Model file for the job. Use its own axes, mm. Face numbers are marked on the shaded views. A direction names the side the tool comes from. Coordinates: 2 decimals unless noted, no trailing zeros. Write each loop counter-clockwise with the first axis right and the second up, starting at its lowest first coordinate (ties: lowest second). Pieces come first, ordered by that corner, then holes. Notation, with made-up numbers: M 83,18.5 L 118,18.5 A19 ccw 118,27.5 Z; hole C 29,-12.5 d2. An arc over 180 degrees is marked long. One line per question, with ' | ' between items. Start each with the question number.
(1) Wall check: probe 1 along Z at (x, y) = (0, 2.25); probe 2 along Z at (x, y) = (0, 3.95); probe 3 along Z at (x, y) = (7, 6.5). Give the ranges that are in metal, low to high.
(2) Cut at D-D (x = -3.25). Write the cut outline in (y, z).
(3) Cut at B-B (z = -11.25). Write the cut outline in (x, y), plus the area to 3 significant figures.
(4) Two-plate mould, pull along X, no slides. Class the marked faces 4, 5 and 6: +X half, -X half, draft (parallel to the pull), parting line (faces both ways), or undercut.
(5) Flat gauge pins, fed straight in: pin 1 Ø3.5 at (x, z) = (-8, 7.5) entering from +Y; pin 2 Ø1 at (x, y) = (8.5, 6.5) entering from -Z; pin 3 Ø4 at (x, z) = (0, 11.11) entering from +Y; pin 4 Ø7.5 at (x, z) = (1, 3.5) entering from -Y. Where does each tip first touch, or does it go through?
(6) Cut at C-C (y = 7.25). Write the cut outline in (x, z) (1 decimal), plus the area to 3 significant figures.
(7) Tool access for the marked faces 1, 2 and 3: list every direction of +Z, -Z, +X, -X, +Y, -Y with a clear straight run to the whole face (end or side of a thin tool).
(8) Cut at A-A (x = 0). Write the cut outline in (y, z).
Autodesk Inventor part; units mm, degrees
ref_plane "a1_XY" through (0, 8.7376, -14.1351) normal (0, 1, 0) x (1, 0, 0)
ref_plane "a1_YZ" through (0, 8.7376, -14.1351) normal (1, 0, 0) x (0, 0, -1)
ref_plane "a1_ZX" through (0, 8.7376, -14.1351) normal (0, 0, -1) x (0, 1, 0)
sketch "Sketch_1" plane through (0, 0, 0) normal (0, 0, 1) x (1, 0, 0)
  line L0 (0, 0) -> (0, 8.7376)
  line L1 (0, 8.7376) -> (14.1351, 8.7376)
  line L2 (14.1351, 8.7376) -> (14.1351, 0)
  line L3 (14.1351, 0) -> (0, 0)
  line L4 (0, 0) -> (0, 8.7376)
revolve "Revolution1" add sketch "Sketch_1" angle 360 about axis through (0, 0, 0) along (0, -1, 0)
sketch "Sketch_63" plane through (0, 0, 0) normal (0, 1, 0) x (-1, 0, 0)
  line L0 (20.6184, 14.1351) -> (13.5509, 14.1351)
  line L1 (13.5509, 14.1351) -> (13.5509, -14.1351)
  line L2 (13.5509, -14.1351) -> (20.6184, -14.1351)
  line L3 (20.6184, -14.1351) -> (20.6184, 14.1351)
extrude "Extrusion1" cut sketch "Sketch_63" along normal blind 8.7376
sketch "Sketch_37" plane through (0, 0, 0) normal (0, 0, 1) x (1, 0, 0)
  line L0 (-5.8778, 4.3688) -> (-14.1351, 4.3688)
  line L1 (-14.1351, 4.3688) -> (-14.1351, 8.3376)
  line L2 (-14.1351, 8.3376) -> (-13.5509, 8.3376)
  line L3 (-13.5509, 8.3376) -> (-13.5509, 6.7818)
  line L4 (-13.5509, 6.7818) -> (-13.1216, 6.3525)
  line L5 (-13.1216, 6.3525) -> (-7.0231, 6.3525)
  line L6 (-7.0231, 6.3525) -> (-5.8778, 4.3688)
  line L7 (-5.8778, 4.3688) -> (-14.1351, 4.3688)
revolve "Revolution2" cut sketch "Sketch_37" angle 360 about axis through (-5.8778, 4.3688, 0) along (1, 0, 0)
thread "Thread1"
sketch "Sketch4" plane through (0, 0, 0) normal (0, -1, 0) x (1, 0, 0)
  point P0 (0, 0)
hole "Hole1" at (0, 0, 0) direction (0, 1, 0) diameter 15.494 depth 2.54
sketch "Sketch5" plane through (0, 8.7376, 0) normal (0, 1, 0) x (1, 0, 0)
  point P0 (0, -11.1125)
hole "Hole2" at (0, 8.7376, 11.1125) direction (0, -1, 0) diameter 3.2639 depth 8.7376 counterbore diameter 4.953 counterbore depth 3.048
sketch "Sketch6" plane through (0, 8.7376, 0) normal (0, 1, 0) x (1, 0, 0)
  point P0 (0, 11.1125)
hole "Hole3" at (0, 8.7376, -11.1125) direction (0, -1, 0) diameter 3.2639 depth 8.7376 counterbore diameter 4.953 counterbore depth 3.048
sketch "Sketch7" plane through (0, 8.7376, 0) normal (0, 1, 0) x (1, 0, 0)
  point P0 (-7.7589, -7.7589)
hole "Hole4" at (-7.7589, 8.7376, 7.7589) direction (0, -1, 0) diameter 2.1565 depth 8.7376 counterbore diameter 3.048 counterbore depth 2.54
pattern_linear "Rectangular Pattern1" count 2 spacing 15.5179 along (1, 0, 0) count 2 spacing 15.5179 along (0, 0, -1) of "Hole4"
ref_plane "a1_XY" through (0, 8.7376, -14.1351) normal (0, 1, 0) x (1, 0, 0)
ref_plane "a1_YZ" through (0, 8.7376, -14.1351) normal (1, 0, 0) x (0, 0, -1)
ref_plane "a1_ZX" through (0, 8.7376, -14.1351) normal (0, 0, -1) x (0, 1, 0)
ref_plane "a2_XY" through (0, 8.7376, 14.1351) normal (0, 1, 0) x (1, 0, 0)
ref_plane "a2_YZ" through (0, 8.7376, 14.1351) normal (1, 0, 0) x (0, 0, -1)
ref_plane "a2_ZX" through (0, 8.7376, 14.1351) normal (0, 0, -1) x (0, 1, 0)
ref_plane "ar3_XY" through (-7.9026, 2.54, 7.9026) normal (0, 1, 0) x (1, 0, 0)
ref_plane "ar3_YZ" through (-7.9026, 2.54, 7.9026) normal (1, 0, 0) x (0, 0, -1)
ref_plane "ar3_ZX" through (-7.9026, 2.54, 7.9026) normal (0, 0, -1) x (0, 1, 0)
ref_plane "ar4_XY" through (7.9026, 2.54, 7.9026) normal (0, 1, 0) x (1, 0, 0)
ref_plane "ar4_YZ" through (7.9026, 2.54, 7.9026) normal (1, 0, 0) x (0, 0, -1)
ref_plane "ar4_ZX" through (7.9026, 2.54, 7.9026) normal (0, 0, -1) x (0, 1, 0)
ref_plane "ar5_XY" through (7.9026, 2.54, -7.9026) normal (0, 1, 0) x (1, 0, 0)
ref_plane "ar5_YZ" through (7.9026, 2.54, -7.9026) normal (1, 0, 0) x (0, 0, -1)
ref_plane "ar5_ZX" through (7.9026, 2.54, -7.9026) normal (0, 0, -1) x (0, 1, 0)
ref_plane "ar6_XY" through (-7.9026, 2.54, -7.9026) normal (0, 1, 0) x (1, 0, 0)
ref_plane "ar6_YZ" through (-7.9026, 2.54, -7.9026) normal (1, 0, 0) x (0, 0, -1)
ref_plane "ar6_ZX" through (-7.9026, 2.54, -7.9026) normal (0, 0, -1) x (0, 1, 0)
ref_plane "b1_XY" through (0, 8.7376, 0) normal (0, 1, 0) x (1, 0, 0)
ref_plane "b1_YZ" through (0, 8.7376, 0) normal (1, 0, 0) x (0, 0, -1)
ref_plane "b1_ZX" through (0, 8.7376, 0) normal (0, 0, -1) x (0, 1, 0)
ref_plane "j_XY" through (0, 0, 0) normal (0, 1, 0) x (1, 0, 0)
ref_plane "j_YZ" through (0, 0, 0) normal (1, 0, 0) x (0, 0, -1)
ref_plane "j_ZX" through (0, 0, 0) normal (0, 0, -1) x (0, 1, 0)
ref_plane "k1_XY" through (-13.5509, 4.3688, 0) normal (0, 0, 1) x (1, 0, 0)
ref_plane "k1_YZ" through (-13.5509, 4.3688, 0) normal (1, 0, 0) x (0, 1, 0)
ref_plane "k1_ZX" through (-13.5509, 4.3688, 0) normal (0, 1, 0) x (0, 0, 1)
ref_plane "k2_XY" through (-13.5509, 8.7376, 0) normal (0, 0, 1) x (1, 0, 0)
ref_plane "k2_YZ" through (-13.5509, 8.7376, 0) normal (1, 0, 0) x (0, 1, 0)
ref_plane "k2_ZX" through (-13.5509, 8.7376, 0) normal (0, 1, 0) x (0, 0, 1)
ref_plane "l1_XY" through (-13.5509, 6.7818, 0) normal (0, 0, 1) x (1, 0, 0)
ref_plane "l1_YZ" through (-13.5509, 6.7818, 0) normal (1, 0, 0) x (0, 1, 0)
ref_plane "l1_ZX" through (-13.5509, 6.7818, 0) normal (0, 1, 0) x (0, 0, 1)
ref_plane "l2_XY" through (-13.5509, 1.9558, 0) normal (0, 0, 1) x (1, 0, 0)
ref_plane "l2_YZ" through (-13.5509, 1.9558, 0) normal (1, 0, 0) x (0, 1, 0)
ref_plane "l2_ZX" through (-13.5509, 1.9558, 0) normal (0, 1, 0) x (0, 0, 1)
ref_plane "po1_XY" through (10.9728, 0, 0) normal (0, 1, 0) x (1, 0, 0)
ref_plane "po1_YZ" through (10.9728, 0, 0) normal (1, 0, 0) x (0, 0, -1)
ref_plane "po1_ZX" through (10.9728, 0, 0) normal (0, 0, -1) x (0, 1, 0)
ref_plane "po2_XY" through (-5.4864, 0, -9.5027) normal (0, 1, 0) x (1, 0, 0)
ref_plane "po2_YZ" through (-5.4864, 0, -9.5027) normal (1, 0, 0) x (0, 0, -1)
ref_plane "po2_ZX" through (-5.4864, 0, -9.5027) normal (0, 0, -1) x (0, 1, 0)
ref_plane "po3_XY" through (-5.4864, 0, 9.5027) normal (0, 1, 0) x (1, 0, 0)
ref_plane "po3_YZ" through (-5.4864, 0, 9.5027) normal (1, 0, 0) x (0, 0, -1)
ref_plane "po3_ZX" through (-5.4864, 0, 9.5027) normal (0, 0, -1) x (0, 1, 0)
ref_plane "r7_XY" through (-1.7526, 8.7376, -11.1125) normal (0, 1, 0) x (1, 0, 0)
ref_plane "r7_YZ" through (-1.7526, 8.7376, -11.1125) normal (1, 0, 0) x (0, 0, -1)
ref_plane "r7_ZX" through (-1.7526, 8.7376, -11.1125) normal (0, 0, -1) x (0, 1, 0)
ref_plane "r71_XY" through (0, 8.7376, 11.1125) normal (0, 1, 0) x (1, 0, 0)
ref_plane "r71_YZ" through (0, 8.7376, 11.1125) normal (1, 0, 0) x (0, 0, -1)
ref_plane "r71_ZX" through (0, 8.7376, 11.1125) normal (0, 0, -1) x (0, 1, 0)
ref_plane "r72_XY" through (1.7526, 8.7376, -11.1125) normal (0, 1, 0) x (1, 0, 0)
ref_plane "r72_YZ" through (1.7526, 8.7376, -11.1125) normal (1, 0, 0) x (0, 0, -1)
ref_plane "r72_ZX" through (1.7526, 8.7376, -11.1125) normal (0, 0, -1) x (0, 1, 0)
ref_plane "r73_XY" through (0, 8.7376, -11.1125) normal (0, 1, 0) x (1, 0, 0)
ref_plane "r73_YZ" through (0, 8.7376, -11.1125) normal (1, 0, 0) x (0, 0, -1)
ref_plane "r73_ZX" through (0, 8.7376, -11.1125) normal (0, 0, -1) x (0, 1, 0)
ref_plane "rg_XY" through (0, 8.7376, 0) normal (0, 1, 0) x (1, 0, 0)
ref_plane "rg_YZ" through (0, 8.7376, 0) normal (1, 0, 0) x (0, 0, -1)
ref_plane "rg_ZX" through (0, 8.7376, 0) normal (0, 0, -1) x (0, 1, 0)
ref_plane "rh_XY" through (0, 8.7376, 0) normal (0, 1, 0) x (1, 0, 0)
ref_plane "rh_YZ" through (0, 8.7376, 0) normal (1, 0, 0) x (0, 0, -1)
ref_plane "rh_ZX" through (0, 8.7376, 0) normal (0, 0, -1) x (0, 1, 0)
ref_plane "rs_1_XY" through (0, 10.5156, -11.1125) normal (0, 1, 0) x (1, 0, 0)
ref_plane "rs_1_YZ" through (0, 10.5156, -11.1125) normal (1, 0, 0) x (0, 0, -1)
ref_plane "rs_1_ZX" through (0, 10.5156, -11.1125) normal (0, 0, -1) x (0, 1, 0)
ref_plane "rs_2_XY" through (-11.1125, 10.5156, 0) normal (0, 1, 0) x (1, 0, 0)
ref_plane "rs_2_YZ" through (-11.1125, 10.5156, 0) normal (1, 0, 0) x (0, 0, -1)
ref_plane "rs_2_ZX" through (-11.1125, 10.5156, 0) normal (0, 0, -1) x (0, 1, 0)
ref_plane "rs_3_XY" through (0, 10.5156, 11.1125) normal (0, 1, 0) x (1, 0, 0)
ref_plane "rs_3_YZ" through (0, 10.5156, 11.1125) normal (1, 0, 0) x (0, 0, -1)
ref_plane "rs_3_ZX" through (0, 10.5156, 11.1125) normal (0, 0, -1) x (0, 1, 0)
ref_plane "rs_4_XY" through (11.1125, 10.5156, 0) normal (0, 1, 0) x (1, 0, 0)
ref_plane "rs_4_YZ" through (11.1125, 10.5156, 0) normal (1, 0, 0) x (0, 0, -1)
ref_plane "rs_4_ZX" through (11.1125, 10.5156, 0) normal (0, 0, -1) x (0, 1, 0)
ref_plane "sc1_XY" through (10.9728, 4.9276, 0) normal (0, 1, 0) x (1, 0, 0)
ref_plane "sc1_YZ" through (10.9728, 4.9276, 0) normal (1, 0, 0) x (0, 0, -1)
ref_plane "sc1_ZX" through (10.9728, 4.9276, 0) normal (0, 0, -1) x (0, 1, 0)
ref_plane "sc2_XY" through (-5.4864, 4.9276, -9.5027) normal (0, 1, 0) x (1, 0, 0)
ref_plane "sc2_YZ" through (-5.4864, 4.9276, -9.5027) normal (1, 0, 0) x (0, 0, -1)
ref_plane "sc2_ZX" through (-5.4864, 4.9276, -9.5027) normal (0, 0, -1) x (0, 1, 0)
ref_plane "sc3_XY" through (-5.4864, 4.9276, 9.5027) normal (0, 1, 0) x (1, 0, 0)
ref_plane "sc3_YZ" through (-5.4864, 4.9276, 9.5027) normal (1, 0, 0) x (0, 0, -1)
ref_plane "sc3_ZX" through (-5.4864, 4.9276, 9.5027) normal (0, 0, -1) x (0, 1, 0)
ref_plane "to_dummy_XY" through (0, 8.7376, 0) normal (0, 1, 0) x (1, 0, 0)
ref_plane "to_dummy_YZ" through (0, 8.7376, 0) normal (1, 0, 0) x (0, 0, -1)
ref_plane "to_dummy_ZX" through (0, 8.7376, 0) normal (0, 0, -1) x (0, 1, 0)
ref_plane "to_nut_XY" through (0, 10.2616, 0) normal (0, 1, 0) x (1, 0, 0)
ref_plane "to_nut_YZ" through (0, 10.2616, 0) normal (1, 0, 0) x (0, 0, -1)
ref_plane "to_nut_ZX" through (0, 10.2616, 0) normal (0, 0, -1) x (0, 1, 0)
ref_plane "to_rod_XY" through (0, 8.7376, 0) normal (0, 1, 0) x (1, 0, 0)
ref_plane "to_rod_YZ" through (0, 8.7376, 0) normal (1, 0, 0) x (0, 0, -1)
ref_plane "to_rod_ZX" through (0, 8.7376, 0) normal (0, 0, -1) x (0, 1, 0)
ref_plane "to_tube_XY" through (0, 2.54, 0) normal (0, 1, 0) x (1, 0, 0)
ref_plane "to_tube_YZ" through (0, 2.54, 0) normal (1, 0, 0) x (0, 0, -1)
ref_plane "to_tube_ZX" through (0, 2.54, 0) normal (0, 0, -1) x (0, 1, 0)
ref_plane "to_wiper_XY" through (0, 8.7376, 0) normal (0, 1, 0) x (1, 0, 0)
ref_plane "to_wiper_YZ" through (0, 8.7376, 0) normal (1, 0, 0) x (0, 0, -1)
ref_plane "to_wiper_ZX" through (0, 8.7376, 0) normal (0, 0, -1) x (0, 1, 0)
ref_plane "track1_XY" through (-7.7851, 0, 0) normal (0, 1, 0) x (1, 0, 0)
ref_plane "track1_YZ" through (-7.7851, 0, 0) normal (1, 0, 0) x (0, 0, -1)
ref_plane "track1_ZX" through (-7.7851, 0, 0) normal (0, 0, -1) x (0, 1, 0)
ref_plane "track2_XY" through (0, 0, -7.7851) normal (0, 1, 0) x (1, 0, 0)
ref_plane "track2_YZ" through (0, 0, -7.7851) normal (1, 0, 0) x (0, 0, -1)
ref_plane "track2_ZX" through (0, 0, -7.7851) normal (0, 0, -1) x (0, 1, 0)
ref_plane "track3_XY" through (7.7851, 0, 0) normal (0, 1, 0) x (1, 0, 0)
ref_plane "track3_YZ" through (7.7851, 0, 0) normal (1, 0, 0) x (0, 0, -1)
ref_plane "track3_ZX" through (7.7851, 0, 0) normal (0, 0, -1) x (0, 1, 0)
ref_plane "track4_XY" through (0, 0, 7.7851) normal (0, 1, 0) x (1, 0, 0)
ref_plane "track4_YZ" through (0, 0, 7.7851) normal (1, 0, 0) x (0, 0, -1)
ref_plane "track4_ZX" through (0, 0, 7.7851) normal (0, 0, -1) x (0, 1, 0)
properties part number "02-2-0.125-FO1_BM_heads_left-bif"
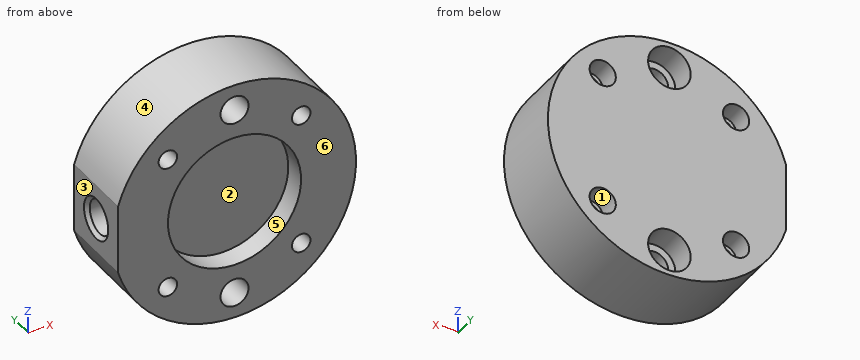
Filled in:
1) probe 1: -14.14 to -12.74, -9.48 to -7.75, 7.75 to 9.48, 12.74 to 14.14 | probe 2: -14.14 to -12.74, -9.48 to 9.48, 12.74 to 14.14 | probe 3: -12.28 to -9.08, -6.44 to 6.44, 9.08 to 12.28
2) outline: M 0,-13.76 L 8.74,-13.76 L 8.74,13.76 L 0,13.76 L 0,7.03 L 2.54,7.03 L 2.54,-7.03 L 0,-7.03 Z
3) outline: M -8.56,0 L -1.63,0 L -1.63,5.69 L -2.47,5.69 L -2.47,8.74 L -8.56,8.74 Z; M 1.63,0 L 8.56,0 L 8.56,8.74 L 2.47,8.74 L 2.47,5.69 L 1.63,5.69 Z | area: 116 mm²
4) face 4: parting line | face 5: undercut | face 6: draft
5) pin 1: y = 8.74 | pin 2: z = -11.65 | pin 3: y = 5.69 | pin 4: y = 2.54
6) outline: M -13.6,-4 A14.1 ccw long -13.6,4 Z; hole C -7.8,-7.8 d3; hole C -7.8,7.8 d3; hole C 0,-11.1 d5; hole C 0,11.1 d5; hole C 7.8,-7.8 d3; hole C 7.8,7.8 d3 | area: 557 mm²
7) face 1: +Y | face 2: -Y | face 3: +Z, -Z, -X, +Y, -Y
8) outline: M 0,-14.14 L 8.74,-14.14 L 8.74,-13.59 L 5.69,-13.59 L 5.69,-12.74 L 0,-12.74 Z; M 0,-9.48 L 5.69,-9.48 L 5.69,-8.64 L 8.74,-8.64 L 8.74,8.64 L 5.69,8.64 L 5.69,9.48 L 0,9.48 L 0,7.75 L 2.54,7.75 L 2.54,-7.75 L 0,-7.75 Z; M 0,12.74 L 5.69,12.74 L 5.69,13.59 L 8.74,13.59 L 8.74,14.14 L 0,14.14 Z
